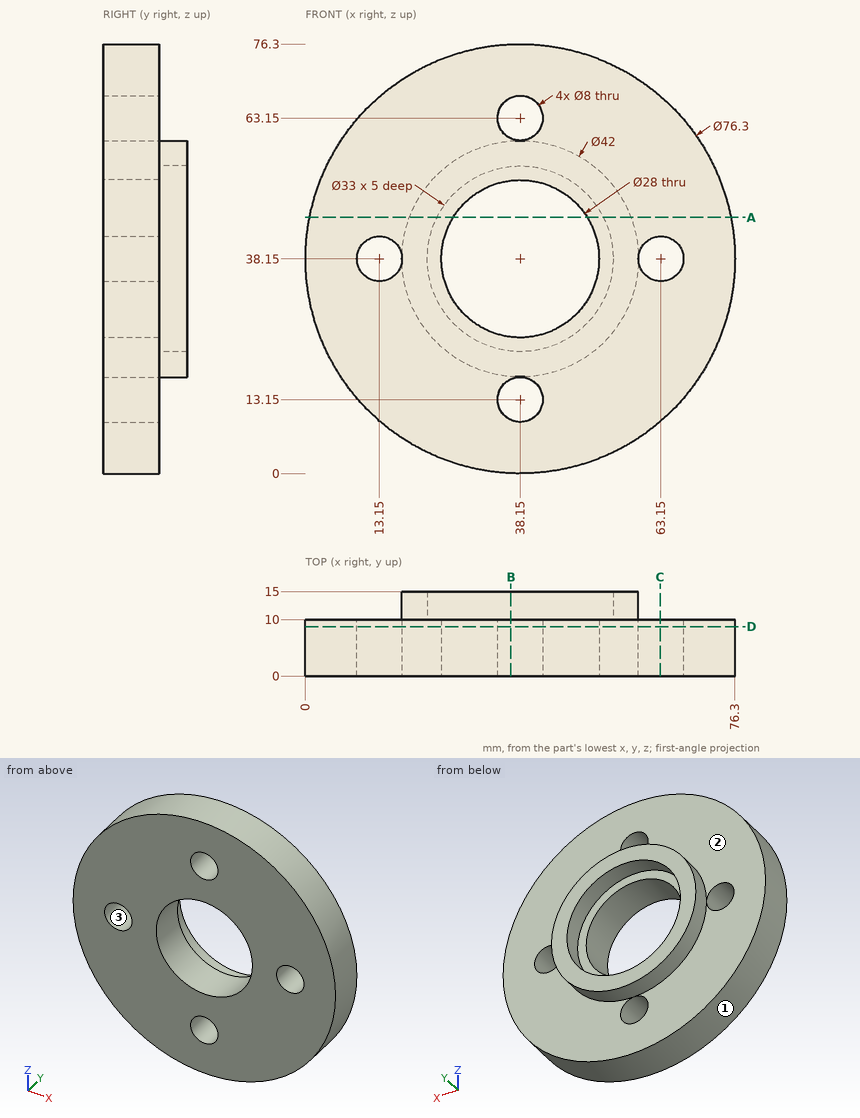
Design review of the part shown in the three views and the two pictorial views. Dimensions are in mm from the part's minimum x, y and z. Round coordinates to 2 decimals unless told otherwise and drop trailing zeros. Write each loop counter-clockwise with the first axis right and the second up, starting at its lowest first coordinate (ties: lowest second). Pieces come first, ordered by that corner, then holes. Notation, with made-up numbers: (-4, 73.5) - (6, 73.5) arc R24 cw to (6, 83.5) - close; hole circle Ø3 at (-16, -40). An arc over 180 degrees is marked (long way). Write item = value, one per line. Start each with the question number.
1. Draft analysis for pull direction X (two halves, no side actions). For the marked faces 1, 2 and 3, state which applies: released by +X, released by -X, zero draft, split by the parting line, or undercut.
2. Consider section B-B on x = 36.5. State the section outline as (y, z) points (1 decimal).
3. Wall thickness on L1, parallel to Z at x = 40, y = 1.5 (1 decimal); L2, parallel to Y at x = 51, z = 48; L3, parallel to X at y = 6.25, z = 48: over which ranges is each line inside the solid? List them lowest first.
4. Consider section D-D on y = 8.75. State the section outline as (x, z) points, plus the area to 3 significant figures.
5. Consider section A-A on z = 45.5. State the section outline as (x, y) points (1 decimal).
6. Consider section C-C on x = 63. State the section outline as (y, z) points, plus the area to 3 significant figures.
7. For pin 1 Ø22.5 at (x, z) = (38.15, 38.15) entering from +Y (3 decimals); pin 2 Ø16.5 at (x, z) = (42, 44) entering from +Y; pin 3 Ø5 at (x, y) = (66, 5) entering from +Z; pin 4 Ø10.5 at (x, z) = (38.15, 63.15) entering from +Y, all flat-tipped, find the tip position at first contact; note any pin that passes through.
Evaluation:
q1.face_1 = split by the parting line
q1.face_2 = zero draft
q1.face_3 = undercut
q2.outline = (0, 0) - (10, 0) - (10, 9.5) - (0, 9.5) - close; (0, 16.8) - (10, 16.8) - (10, 17.2) - (15, 17.2) - (15, 21.7) - (10, 21.7) - (10, 24.2) - (0, 24.2) - close; (0, 52.1) - (10, 52.1) - (10, 54.6) - (15, 54.6) - (15, 59.1) - (10, 59.1) - (10, 59.5) - (0, 59.5) - close; (0, 66.8) - (10, 66.8) - (10, 76.3) - (0, 76.3) - close
q3.L1 = 0 to 9.6, 16.7 to 24.3, 52 to 59.6, 66.7 to 76.3
q3.L2 = 0 to 10
q3.L3 = 1.29 to 28.2, 48.1 to 75.01
q4.outline = circle Ø76.3 at (38.15, 38.15); hole circle Ø8 at (13.15, 38.15); hole circle Ø28 at (38.15, 38.15); hole circle Ø8 at (38.15, 13.15); hole circle Ø8 at (38.15, 63.15); hole circle Ø8 at (63.15, 38.15)
q4.area = 3,760 mm2
q5.outline = (0.7, 0) - (26.2, 0) - (26.2, 10) - (23.4, 10) - (23.4, 15) - (18.5, 15) - (18.5, 10) - (0.7, 10) - close; (50.1, 0) - (75.6, 0) - (75.6, 10) - (57.8, 10) - (57.8, 15) - (52.9, 15) - (52.9, 10) - (50.1, 10) - close
q6.outline = (0, 9.2) - (10, 9.2) - (10, 34.15) - (0, 34.15) - close; (0, 42.15) - (10, 42.15) - (10, 67.1) - (0, 67.1) - close
q6.area = 499 mm2
q7.pin_1 = through
q7.pin_2 = 10
q7.pin_3 = 66.66
q7.pin_4 = 15
